Check sheet for the drawn part. Datum: minimum x, y, z corner. Units: mm. Round coordinates to 2 decimals unless told otherwise and drop trailing zeros. Write each loop counter-clockwise with the first axis right and the second up, starting at its lowest first coordinate (ties: lowest second). Pieces come first, ordered by that corner, then holes.
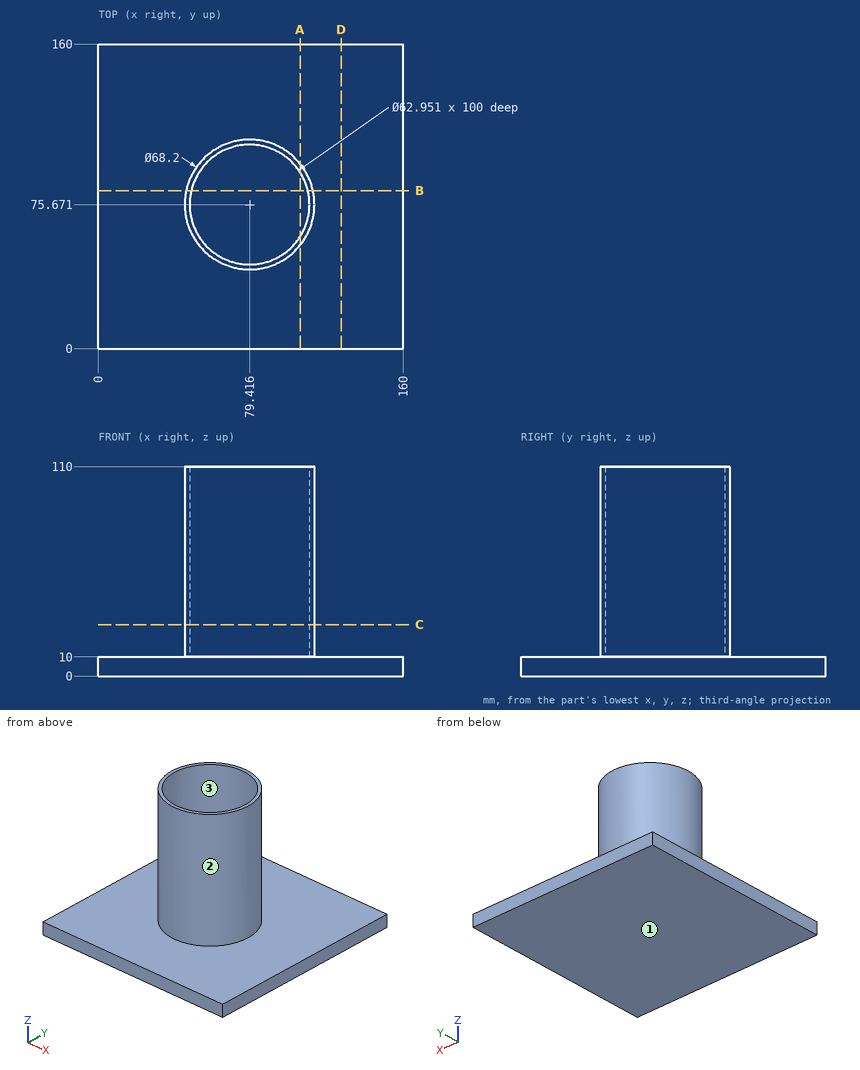
1. Sectioned sample at C-C, the plane z = 27. Enter the section's corners in (x, y) (1 decimal).
2. Sectioned sample at B-B, the plane y = 83. Enter the section's corners in (x, z).
3. Sectioned sample at A-A, the plane x = 106. Enter the section's corners in (y, z) (1 decimal), plus the area to 3 significant figures.
4. Go/stop test with flat-tipped pins: pin 1 (2 mm diameter, centred on x = 137.5, y = 95.5, fed in from +Z); pin 2 (8 mm diameter, centred on y = 76.5, z = 80, fed in from +X); pin 3 (6 mm diameter, centred on x = 84, z = 17.5, fed in from +Y). Record where each tip stops, or that it passes through.
5. Sectioned sample at D-D, the plane x = 127.5. Enter the section's corners in (y, z), plus the area to 3 significant figures.
6. Scan lines: line 1 along X through (y, z) = (74, 91) (1 decimal); line 2 along Z through (x, y) = (81, 153.5); line 3 along Y through (x, z) = (84.5, 73.5). Record each from-to range of solid material in increasing order.
7. Release check for a two-part mould opening along X. For the marked faces 1, 2 and 3 record: released by +X, released by -X, zero draft, split by the parting line, or undercut.
Computed values:
1. outline: circle Ø68.2 at (79.4, 75.7); hole circle Ø63 at (79.4, 75.7)
2. outline: (0, 0) - (160, 0) - (160, 10) - (112.72, 10) - (112.72, 110) - (110.03, 110) - (110.03, 10) - (48.81, 10) - (48.81, 110) - (46.11, 110) - (46.11, 10) - (0, 10) - close
3. outline: (0, 0) - (160, 0) - (160, 10) - (97, 10) - (97, 110) - (92.5, 110) - (92.5, 10) - (58.8, 10) - (58.8, 110) - (54.3, 110) - (54.3, 10) - (0, 10) - close
3. area: 2,500 mm2
4. pin 1: stops at z = 10
4. pin 2: stops at x = 113.52
4. pin 3: stops at y = 109.73
5. outline: (0, 0) - (160, 0) - (160, 10) - (0, 10) - close
5. area: 1,600 mm2
6. line 1: x = 45.4 to 48, 110.8 to 113.5
6. line 2: z = 0 to 10
6. line 3: y = 41.95 to 44.61, 106.73 to 109.39
7. face 1: zero draft
7. face 2: split by the parting line
7. face 3: undercut
